The figure shows three views and two pictorial views of one solid part (mm, origin at its lowest corner). Answer the questions. A direction names the side the tool comes from. Coordinates: 2 decimals unless noted, no trailing zeros. Loops run counter-clockwise (first coordinate to the right, second up) from the corner with the lowest first, then second, coordinate; pieces in that order, holes last.
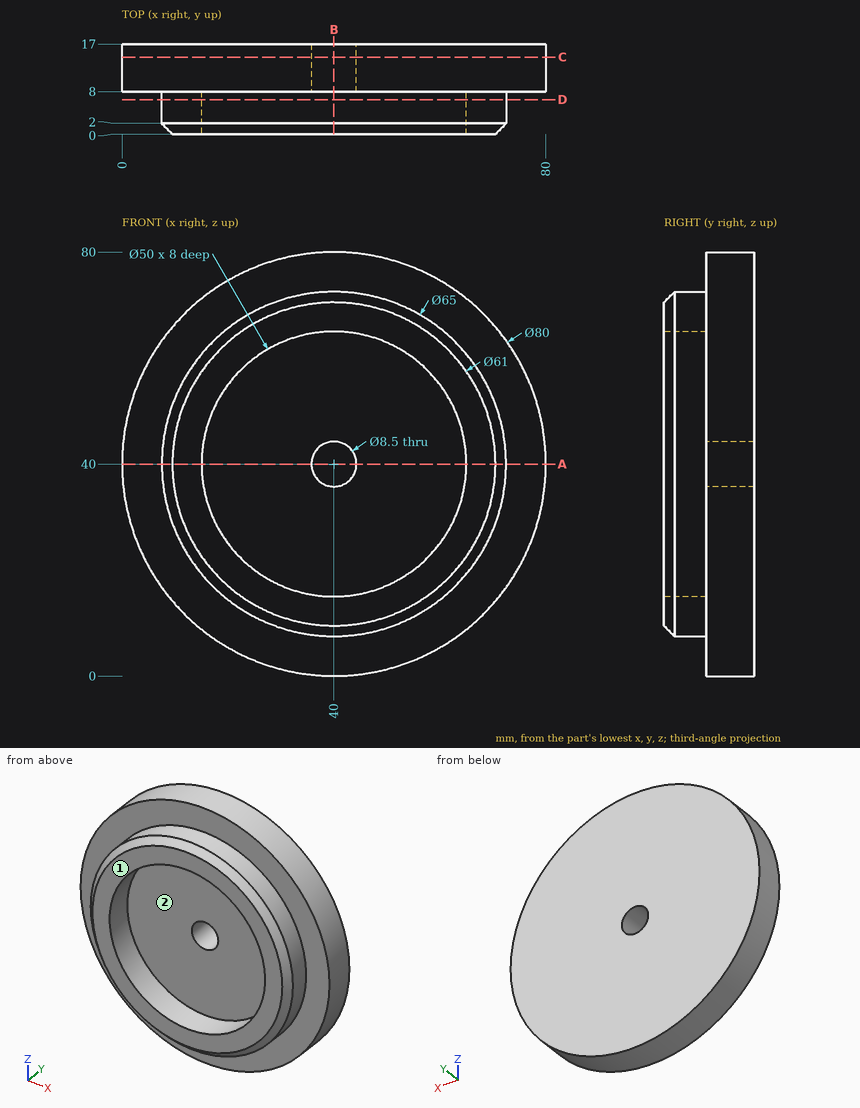
1. Each of these flat-tipped pins is pushed along its axis until it touches: P1, Ø2, axis at y = 4, z = 23.5, coming from the +X side; P2, Ø25, axis at x = 32, z = 49, coming from the -Y side; P3, Ø10, axis at y = 11, z = 56.5, coming from the -X side; P4, Ø7, axis at x = 40, z = 40, coming from the -Y side. Where does it stop, or does it pass through?
2. A cutting plane is placed at A-A, the plane z = 40. Give the vertices of the cut face in (x, y).
3. Straight lines are drawn through the part: probe 1 along Z at (x, y) = (40, 4.75); probe 2 along Z at (x, y) = (40, 12.5); probe 3 along Y at (x, z) = (19.5, 71). For each, find the intervals that lie inside material, in ascending order.
4. A cutting plane is placed at D-D, the plane y = 6.5. Give the vertices of the cut face in (x, z).
5. A cutting plane is placed at B-B, the plane x = 40. Give the vertices of the cut face in (y, z).
6. For the marked faces 1 and 2, determine the directions among +Z, -Z, +X, -X, +Y, -Y from which every point of the face is accessible in a straight line to the end or side of a thin tool.
7. A cutting plane is placed at C-C, the plane y = 14.5. Give the vertices of the cut face in (x, z).
Answers below:
1. P1: stops at x = 68.57
1. P2: stops at y = 8
1. P3: stops at x = 1.69
1. P4: passes through
2. outline: (0, 8) - (7.5, 8) - (7.5, 2) - (9.5, 0) - (15, 0) - (15, 8) - (35.75, 8) - (35.75, 17) - (0, 17) - close; (44.25, 8) - (65, 8) - (65, 0) - (70.5, 0) - (72.5, 2) - (72.5, 8) - (80, 8) - (80, 17) - (44.25, 17) - close
3. probe 1: z = 7.5 to 15, 65 to 72.5
3. probe 2: z = 0 to 35.75, 44.25 to 80
3. probe 3: y = 8 to 17
4. outline: circle Ø65 at (40, 40); hole circle Ø50 at (40, 40)
5. outline: (0, 9.5) - (2, 7.5) - (8, 7.5) - (8, 0) - (17, 0) - (17, 35.75) - (8, 35.75) - (8, 15) - (0, 15) - close; (0, 65) - (8, 65) - (8, 44.25) - (17, 44.25) - (17, 80) - (8, 80) - (8, 72.5) - (2, 72.5) - (0, 70.5) - close
6. face 1: +Z, -Z, +X, -X, -Y
6. face 2: -Y
7. outline: circle Ø80 at (40, 40); hole circle Ø8.5 at (40, 40)
